Part model, mm, in its own coordinate system. A direction names the side the tool comes from. Give positions to 0.01 mm unless a question says otherwise; leave off trailing zeros. Order: outer loops, then holes, each group sorted by start corner. A loop starts at its lowest first (then second) coordinate and runs counter-clockwise, first axis right, second up. Notation, with made-up numbers: M -1,74 L 9,74 A23 ccw 9,109 Z; hole C 69.25,22 d1. An arc over 180 degrees is marked long. Return JSON: item names as keys, results as strings.
Autodesk Inventor part; units mm, degrees
ref_plane "YZ Plane" through (0, 0, 0) normal (1, 0, 0) x (0, 1, 0)
ref_plane "XZ Plane" through (0, 0, 0) normal (0, 1, 0) x (-1, 0, 0)
ref_plane "XY Plane" through (0, 0, 0) normal (0, 0, 1) x (1, 0, 0)
sketch "Sketch1" plane through (0, 0, 0) normal (0, 1, 0) x (-1, 0, 0)
  line L0 (73.75, -5.35) -> (61.25, -5.35)
  line L1 (61.25, -5.35) -> (61.25, -17.85)
  line L2 (61.25, -17.85) -> (73.75, -17.85)
  line L3 (73.75, -17.85) -> (73.75, -5.35)
  line L4 (107.5984, -0.1) -> (40.7, -0.1)
  line L5 (40.7, -23.1) -> (107.5984, -23.1)
  line L6 (77.3838, -11.6) -> (49.3838, -11.6) construction
  line L7 (67.5, -2.25) -> (67.5, -23.25) construction
  line L8 (101.5, -0.1) -> (101.5, -23.1)
  line L9 (103.3, -23.1) -> (103.3, -0.1)
  line L10 (81.5, -9.1) -> (107.5984, -9.1)
  line L11 (107.5984, -14.1) -> (81.5, -14.1)
  line L12 (48.5, -23.1) -> (48.5, -0.1)
  line L13 (46.7, -0.1) -> (46.7, -23.1)
  line L14 (53.5, -10.1) -> (40.7, -10.1)
  line L15 (53.5, -13.1) -> (40.7, -13.1)
  line L16 (101.5, -15.5) -> (100, -15.5)
  line L17 (100, -15.5) -> (100, -7.7)
  line L18 (100, -7.7) -> (101.5, -7.7)
  line L19 (79.5, -0.1) -> (79.5, -23.1)
  line L20 (81.5, -23.1) -> (81.5, -0.1)
  line L21 (55.5, -0.1) -> (55.5, -23.1)
  line L22 (53.5, -23.1) -> (53.5, -0.1)
  line L23 (79.5, -13.1) -> (73.75, -13.1)
  line L24 (73.75, -10.1) -> (79.5, -10.1)
  line L25 (61.25, -13.1) -> (55.5, -13.1)
  line L26 (55.5, -10.1) -> (61.25, -10.1)
  line L27 (73.75, -17.85) -> (77.95, -17.85)
  line L28 (77.95, -17.85) -> (77.95, -14.65)
  line L29 (77.95, -14.65) -> (73.75, -14.65)
  line L30 (73.75, -14.65) -> (61.25, -14.65)
  line L31 (56.65, -14.65) -> (56.65, -17.85)
  line L32 (56.65, -17.85) -> (59.85, -17.85)
  line L33 (59.85, -14.65) -> (56.65, -14.65)
  line L34 (59.85, -5.35) -> (56.65, -5.35)
  line L35 (56.65, -5.35) -> (56.65, -8.55)
  line L36 (56.65, -8.55) -> (59.85, -8.55)
  line L37 (61.25, -8.55) -> (73.75, -8.55)
  line L38 (77.95, -8.55) -> (77.95, -5.35)
  line L39 (73.75, -5.35) -> (77.95, -5.35)
  line L40 (77.95, -8.55) -> (73.75, -8.55)
  line L41 (59.85, -17.85) -> (59.85, -14.65)
  line L42 (59.85, -8.55) -> (59.85, -5.35)
  line L43 (61.25, -17.85) -> (59.85, -17.85)
  line L44 (61.25, -14.65) -> (59.85, -14.65)
  line L45 (61.25, -8.55) -> (59.85, -8.55)
  line L46 (61.25, -5.35) -> (59.85, -5.35)
  line L47 (40.7, -23.1) -> (40.7, -0.1)
  line L48 (107.5984, -23.1) -> (107.5984, -0.1)
  point P0 (103.3, -9.1)
  point P1 (101.5, -9.1)
  point P2 (103.3, -14.1)
  point P3 (101.5, -14.1)
  point P4 (48.5, -10.1)
  point P5 (46.7, -10.1)
  point P6 (48.5, -13.1)
  point P7 (46.7, -13.1)
  point P8 (67.5, -11.6)
  point P9 (100, -9.1)
  point P10 (100, -14.1)
  dimension "d0" = 12.5
  dimension "d1" = 12.5
  dimension "d7" = 1.8
  dimension "d12" = 5
  dimension "d18" = 1.8
  dimension "d39" = 1.5
  dimension "d43" = 2
  dimension "d45" = 2
  dimension "d52" = 12
  dimension "d57" = 12
  dimension "d62" = 3
  dimension "d63" = 3
  dimension "d67" = 22
  dimension "d71" = 7
  dimension "d76" = 4.2
  dimension "d77" = 3.2
  dimension "d78" = 3.2
  dimension "d79" = 1.4
  dimension "d80" = 3.2
  dimension "d91" = 6
  dimension "d92" = 3
  dimension "d95" = 23
extrude "Extrusion11" add sketch "Sketch1" against normal blind 3 contours L3 L37 L1 L0 | L1 L45 L42 L46 | L3 L2 L1 L30 | L1 L43 L41 L44
extrude "Extrusion10" add sketch "Sketch1" against normal blind 6 separate body contours L0 L46 L34 L35 L36 L45 L1 L26 L21 L4 L19 L24 L3 L40 L38 L39 | L3 L30 L1 L37 | L24 L19 L23 L3 | L1 L25 L21 L26 | L23 L19 L5 L21 L25 L1 L44 L33 L31 L32 L43 L2 L27 L28 L29 L3 | L19 L4 L20 L5 | L21 L5 L22 L4 | L4 L8 L18 L17 L10 L20 | L22 L14 L12 L4 | L20 L11 L17 L16 L8 L5 | L4 L9 L10 L8 | L10 L17 L11 L20 | L5 L12 L15 L22 | L12 L14 L13 L4 | L22 L15 L12 L14 | L8 L11 L9 L5 | L4 L48 L10 L9 | L8 L10 L17 L18 | L10 L8 L11 L17 | L5 L13 L15 L12 | L13 L14 L47 L4 | L12 L15 L13 L14 | L9 L11 L48 L5 | L16 L17 L11 L8 | L10 L48 L11 L9 | L9 L11 L8 L10 | L5 L47 L15 L13 | L13 L15 L47 L14
extrude "Extrusion15" add sketch "Sketch1" along normal blind 5 contours L0 L46 L34 L35 L36 L45 L1 L26 L21 L4 L19 L24 L3 L40 L38 L39 | L24 L19 L23 L3 | L1 L25 L21 L26 | L23 L19 L5 L21 L25 L1 L44 L33 L31 L32 L43 L2 L27 L28 L29 L3 | L4 L8 L18 L17 L10 L20 | L22 L14 L12 L4 | L20 L11 L17 L16 L8 L5 | L10 L17 L11 L20 | L5 L12 L15 L22 | L22 L15 L12 L14 | L4 L48 L10 L9 | L8 L10 L17 L18 | L10 L8 L11 L17 | L13 L14 L47 L4 | L9 L11 L48 L5 | L16 L17 L11 L8 | L10 L48 L11 L9 | L5 L47 L15 L13 | L13 L15 L47 L14
extrude "Extrusion14" add sketch "Sketch1" along normal blind 3.5 contours L3 L37 L1 L0 | L3 L30 L1 L37 | L3 L2 L1 L30
extrude "Extrusion16" add sketch "Sketch1" along normal blind 20 contours L0 L46 L34 L35 L36 L45 L1 L26 L21 L4 L19 L24 L3 L40 L38 L39 | L1 L45 L42 L46 | L23 L19 L5 L21 L25 L1 L44 L33 L31 L32 L43 L2 L27 L28 L29 L3 | L1 L43 L41 L44 | L4 L8 L18 L17 L10 L20 | L22 L14 L12 L4 | L20 L11 L17 L16 L8 L5 | L5 L12 L15 L22 | L4 L48 L10 L9 | L13 L14 L47 L4 | L9 L11 L48 L5 | L5 L47 L15 L13
properties part number "Spirulina_prototype"
Q1. Band-saw the part on A-A (z = -6.25). Give the number of separate pieces and of enclosed holes in the cut face, then the cut area to 3 significant figures.
Established:
{"separate pieces": "3", "enclosed holes": "0", "area": "1,150 mm²"}
Q2. Band-saw the part on D-D (z = -11). Give the cut face in (x, y).
Established:
{"outline": "M -107.6,-6 L -40.7,-6 L -40.7,5 L -46.7,5 L -46.7,0 L -48.5,0 L -48.5,5 L -53.5,5 L -53.5,0 L -55.5,0 L -55.5,5 L -61.25,5 L -61.25,3.5 L -73.75,3.5 L -73.75,5 L -79.5,5 L -79.5,0 L -81.5,0 L -81.5,5 L -101.5,5 L -101.5,0 L -103.3,0 L -103.3,5 L -107.6,5 Z"}
Q3. Two-plate mould, pull along Z, no slides. Class faces 1 (the flat face through (-91, 20, -19)), 2 (the flat face through (-67, 7, -5.35)): +Z half, -Z half, draft (parallel to the pull), parting line (faces both ways), or undercut.
Established:
{"face 1": "draft", "face 2": "undercut"}
Q4. Pin check, flat tips, straight feed: pin 1 (10 mm diameter, centred on y = 7.5, z = -11.5, fed in from +X); pin 2 (3 mm diameter, centred on y = 17, z = -12.5, fed in from -X). Stop position of each tip, or through.
Established:
{"pin 1": "stops at x = -40.7", "pin 2": "stops at x = -79.5"}
Q5. Band-saw the part on C-C (x = -62.5). Give the cut face in (y, z), then the cut area to 3 significant figures.
Established:
{"outline": "M -6,-23.1 L 20,-23.1 L 20,-17.85 L 3.5,-17.85 L 3.5,-5.35 L 20,-5.35 L 20,-0.1 L -6,-0.1 L -6,-5.35 L -3,-5.35 L -3,-8.55 L -6,-8.55 L -6,-14.65 L -3,-14.65 L -3,-17.85 L -6,-17.85 Z", "area": "373 mm²"}
Q6. Probe line 1 along Z through (x, y) = (-76.5, -4); line 2 along X through (y, z) = (7, -2); line 3 along Z through (x, y) = (-75, 8.75). List the from-to ranges inside material, lowest first.
Established:
{"line 1": "z = -23.1 to -17.85, -14.65 to -8.55, -5.35 to -0.1", "line 2": "x = -107.6 to -103.3, -101.5 to -81.5, -79.5 to -55.5, -53.5 to -48.5, -46.7 to -40.7", "line 3": "z = -23.1 to -17.85, -14.65 to -13.1, -10.1 to -8.55, -5.35 to -0.1"}
Q7. 3-axis set-ups, long thin cutter, end or side, ignore diameter. For faces 3 (the flat face through (-73.75, 12, -14)), 4 (the flat face through (-77, 12, -13.1)), 5 (the flat face through (-67, -3, -16)), 6 (the flat face through (-77.95, 7, -16)): which of +Z, -Z, +X, -X, +Y, -Y reach the whole face in a straight line?
Established:
{"face 3": "+Y", "face 4": "+X, -X, +Y", "face 5": "-Y", "face 6": "+Y, -Y"}
